Verification items for the finished model (mm, model axes). A direction names the side the tool comes from. Coordinates: 2 decimals unless noted, no trailing zeros. Write each loop counter-clockwise with the first axis right and the second up, starting at its lowest first coordinate (ties: lowest second). Pieces come first, ordered by that corner, then holes. Notation, with made-up numbers: M -13,-23 L 22,-23 A24 ccw 22,-11 Z; hole C 47,47.5 d10. An arc over 180 degrees is marked long. Answer in a Markdown table with one row per item.
from build123d import *

# Parameters (mm, degrees)
SKETCH1_R           = 2.5
SKETCH1_R_2         = 45
SKETCH1_R_3         = 4
BOSS_EXTRUDE1_DEPTH = 5
SKETCH2_R           = 3
BOSS_EXTRUDE3_DEPTH = 5


with BuildPart() as part:
    # Sketch1 → Boss-Extrude1 (new body)
    with BuildSketch(Plane.XY):
        with BuildLine():
            Line((-303.125, -24.803918541), (-7.8125, -62.009796353))
            ThreePointArc((-7.8125, -62.009796353), (62.5, 0), (-7.8125, 62.009796353))
            Line((-7.8125, 62.009796353), (-303.125, 24.803918541))
            ThreePointArc((-303.125, 24.803918541), (-325, 0), (-303.125, -24.803918541))
        make_face()
        with Locations((-220, -7.5)):
            Circle(SKETCH1_R, mode=Mode.SUBTRACT)
        with Locations((-90, -7.5)):
            Circle(SKETCH1_R, mode=Mode.SUBTRACT)
        with Locations((-220, 7.5)):
            Circle(SKETCH1_R, mode=Mode.SUBTRACT)
        with Locations((-155, 0)):
            Circle(SKETCH1_R, mode=Mode.SUBTRACT)
        with Locations((-90, 7.5)):
            Circle(SKETCH1_R, mode=Mode.SUBTRACT)
        with Locations((39, 39)):
            Circle(SKETCH1_R, mode=Mode.SUBTRACT)
        with Locations((-39, -39)):
            Circle(SKETCH1_R, mode=Mode.SUBTRACT)
        with Locations((39, -39)):
            Circle(SKETCH1_R, mode=Mode.SUBTRACT)
        Circle(SKETCH1_R_2, mode=Mode.SUBTRACT)
        with Locations((-39, 39)):
            Circle(SKETCH1_R, mode=Mode.SUBTRACT)
        with Locations((-300, 0)):
            Circle(SKETCH1_R_3, mode=Mode.SUBTRACT)
    extrude(amount=BOSS_EXTRUDE1_DEPTH)

    # Sketch2 → Boss-Extrude3 (add)
    with BuildSketch(Plane(origin=(0, 0, 0), x_dir=(-1, 0, 0), z_dir=(0, 0, -1))):
        Polygon((-62.5, 0), (-91.073673697, 21.751815091), (-55.889899017, 67.970013109), (-22.218770371, 58.417259806), (-51.948744274, 34.750222566), align=None)
        with Locations((-54.840808576, 57.745505577)):
            Circle(SKETCH2_R, mode=Mode.SUBTRACT)
        with Locations((-82.098001573, 21.939843596)):
            Circle(SKETCH2_R, mode=Mode.SUBTRACT)
    extrude(amount=-BOSS_EXTRUDE3_DEPTH)


solid = part.part
1) Sectioned sample at D-D (x = -246). Record the cut outline in (y, z), then the cut area to 3 significant figures.
Response values:
| item | result |
|---|---|
| outline | M -32,0 L 32,0 L 32,5 L -32,5 Z |
| area | 320 mm² |
2) Thickness scan on L1, parallel to Y at x = 0, z = 2.2; L2, parallel to Y at x = -153.5, z = 4.7; L3, parallel to X at y = 1.5, z = 4.5 (3 decimals). Record the ranges inside material, lowest first. Write a range as [from, to].
Response values:
| item | result |
|---|---|
| L1 | y = [-62.5, -45], [45, 62.5] |
| L2 | y = [-43.65, -2], [2, 43.65] |
| L3 | x = [-324.955, -303.708], [-296.292, -157], [-153, -44.975], [44.975, 64.47] |
3) Sectioned sample at B-B (z = 1.45). Give the number of separate pieces and of enclosed holes in the cut face, then the cut area to 3 significant figures.
Response values:
| item | result |
|---|---|
| separate pieces | 1 |
| enclosed holes | 13 |
| area | 28,600 mm² |
4) Sectioned sample at A-A (x = 0). Record the cut outline in (y, z), then the cut area to 3 significant figures.
Response values:
| item | result |
|---|---|
| outline | M -62.5,0 L -45,0 L -45,5 L -62.5,5 Z; M 45,0 L 62.5,0 L 62.5,5 L 45,5 Z |
| area | 175 mm² |
5) Sectioned sample at C-C (x = -142.5). Record the cut outline in (y, z).
Response values:
| item | result |
|---|---|
| outline | M -45.04,0 L 45.04,0 L 45.04,5 L -45.04,5 Z |
6) Depth check by flat-ended pin: pin 1 (1 mm diameter, centred on x = -92, y = 6.5, fed in from +Z); pin 2 (1.5 mm diameter, centred on x = 22, z = 3, fed in from +Y). Enter the tip coordinate at first touch or a pass-through.
Response values:
| item | result |
|---|---|
| pin 1 | stops at z = 5 |
| pin 2 | stops at y = 58.78 |
7) Tool access check on faces 1 (the face through (39.29, 63.26, 2.46)), 2 (the face through (-153.402, 43.667, 2.465)). Record the directions out of +Z, -Z, +X, -X, +Y, -Y that give a thin tool (end or side, any length) a straight path to the whole face; none if there is none.
Response values:
| item | result |
|---|---|
| face 1 | +Z, -Z, +Y |
| face 2 | +Z, -Z, -X, +Y |
8) Release check for a two-part mould opening along X. For faces 3 (the face through (-120, 4, 0)), 4 (the face through (-304, 0, 2)), 5 (the face through (-157.536, -43.146, 2.465)) record: +X half, -X half, draft (parallel to the pull), parting line (faces both ways), or undercut.
Response values:
| item | result |
|---|---|
| face 3 | draft |
| face 4 | undercut |
| face 5 | -X half |
